from build123d import *

# Parameters (mm, degrees)
BOSS_EXTRUDE1_DEPTH = 50
SHELL1_T            = -1.5
SKETCH2_R           = 2.5
CUT_EXTRUDE1_DEPTH  = 50
SKETCH3_OUTSIDE_W   = 127.464
SKETCH3_OUTSIDE_H   = 87.464
CUT_EXTRUDE2_DEPTH  = 5
CUT_EXTRUDE2_TAPER  = 0.5
FILLET1_R           = 0.5
CHAMFER1_SIZE       = 1.25


with BuildPart() as part:
    # Sketch1 → Boss-Extrude1 (new body)
    with BuildSketch(Plane(origin=(0, 0, 0), x_dir=(1, 0, 0), z_dir=(0, 1, 0))):
        with BuildLine():
            Line((-47.5, -30), (47.5, -30))
            ThreePointArc((47.5, -30), (49.267766953, -29.267766953), (50, -27.5))
            Line((50, -27.5), (50, 27.5))
            ThreePointArc((50, 27.5), (49.267766953, 29.267766953), (47.5, 30))
            Line((47.5, 30), (-47.5, 30))
            ThreePointArc((-47.5, 30), (-49.267766953, 29.267766953), (-50, 27.5))
            Line((-50, 27.5), (-50, -27.5))
            ThreePointArc((-50, -27.5), (-49.267766953, -29.267766953), (-47.5, -30))
        make_face()
    extrude(amount=BOSS_EXTRUDE1_DEPTH)

    # Shell1
    shell1_openings = [part.faces().sort_by_distance(p)[0] for p in [
        (0, 50, 0),
    ]]
    offset(amount=SHELL1_T, openings=shell1_openings, kind=Kind.INTERSECTION)

    # Sketch2 → Cut-Extrude1 (cut)
    with BuildSketch(Plane(origin=(0, 1.5, 0), x_dir=(1, 0, 0), z_dir=(0, 1, 0))):
        with Locations((-40, 20)):
            Circle(SKETCH2_R)
        with Locations((40, 20)):
            Circle(SKETCH2_R)
        with Locations((40, -20)):
            Circle(SKETCH2_R)
        with Locations((-40, -20)):
            Circle(SKETCH2_R)
    extrude(amount=-CUT_EXTRUDE1_DEPTH, mode=Mode.SUBTRACT)

    # Sketch3 outside → Cut-Extrude2 (cut)
    with BuildSketch(Plane(origin=(0, 50, 0), x_dir=(1, 0, 0), z_dir=(0, 1, 0))):
        Rectangle(SKETCH3_OUTSIDE_W, SKETCH3_OUTSIDE_H)
        with BuildLine():
            Line((-47.767766953, -29.267766953), (47.767766953, -29.267766953))
            ThreePointArc((47.767766953, -29.267766953), (48.828427125, -28.828427125), (49.267766953, -27.767766953))
            Line((49.267766953, -27.767766953), (49.267766953, 27.767766953))
            ThreePointArc((49.267766953, 27.767766953), (48.828427125, 28.828427125), (47.767766953, 29.267766953))
            Line((47.767766953, 29.267766953), (-47.767766953, 29.267766953))
            ThreePointArc((-47.767766953, 29.267766953), (-48.828427125, 28.828427125), (-49.267766953, 27.767766953))
            Line((-49.267766953, 27.767766953), (-49.267766953, -27.767766953))
            ThreePointArc((-49.267766953, -27.767766953), (-48.828427125, -28.828427125), (-47.767766953, -29.267766953))
        make_face(mode=Mode.SUBTRACT)
    extrude(amount=-CUT_EXTRUDE2_DEPTH, taper=CUT_EXTRUDE2_TAPER, mode=Mode.SUBTRACT)

    # Fillet1
    fillet1_edges = [part.edges().sort_by_distance(p)[0] for p in [
        (-50, 0, 0),
        (-49.267766953, 0, -29.267766953),
        (0, 0, -30),
        (49.267766953, 0, -29.267766953),
        (50, 0, 0),
        (49.267766953, 0, 29.267766953),
        (0, 0, 30),
        (-49.267766953, 0, 29.267766953),
    ]]
    fillet(fillet1_edges, radius=FILLET1_R)

    # Chamfer1
    chamfer1_edges = [part.edges().sort_by_distance(p)[0] for p in [
        (-42.5, 1.5, -20),
        (37.5, 1.5, -20),
        (37.5, 1.5, 20),
        (-42.5, 1.5, 20),
    ]]
    chamfer(chamfer1_edges, length=CHAMFER1_SIZE)


solid = part.part
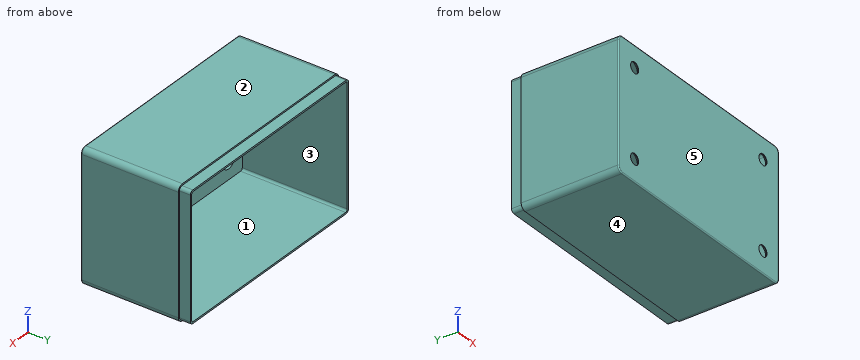
Read the model definition and answer for the solid it produces. Units are mm, in the model's axes. Face numbers are marked on the shaded views. A direction names the side the tool comes from. Give positions to 0.01 mm unless a question says otherwise; leave off trailing zeros. Loops run counter-clockwise (first coordinate to the right, second up) from the corner with the lowest first, then second, coordinate; pieces in that order, holes last. Notation, with made-up numbers: (50.25, -19.75) - (88.25, -19.75) arc R10 cw to (88.25, -1.75) - close; hole circle Ø4 at (38, -9). An arc over 180 degrees is marked (long way). Answer as CSV lines item,"result". Start each with the question number.
1) Which of the six approach directions +Z, -Z, +X, -X, +Y, -Y give full straight-line access (tool end or side, diameter ignored) to the marked faces 1 and 2?
2) Straight lines are drawn through the part: L1, parallel to X at y = 24.5, z = 23; L2, parallel to Z at x = 2, y = 28; L3, parallel to Z at x = 40, y = 0.1. For each, find the intervals that lie inside material, in ascending order. Write a range as from..to.
3) Find section B-B (x = -40). State how many separate pieces and enclosed holes the cut face has, then the cut area to 3 significant figures.
4) Find section A-A (y = 10). Write down the section's boundary in (x, z), then the cut area to 3 significant figures.
5) Determine the mould class of the marked faces 3, 4 and 5 for opening direction Z: released by +Z, released by -Z, zero draft, split by the parting line, or undercut.
6) Each of these flat-tipped pins is pushed along its axis until it touches: pin 1 Ø6.5 at (x, z) = (40, 20) entering from -Y; pin 2 Ø18 at (x, z) = (-9, -3.5) entering from +Y. Where does it stop, or does it pass through?
Findings below:
1,face 1,"+Y"
1,face 2,"+Z, +X, -X, +Y, -Y"
2,L1,"-50..-48.5, 48.5..50"
2,L2,"-30..-28.5, 28.5..30"
2,L3,"-29.8..-22.5, -17.5..17.5, 22.5..29.8"
3,separate pieces,"3"
3,enclosed holes,"0"
3,area,"210 mm^2"
4,outline,"(-50, -27.5) arc R2.5 ccw to (-47.5, -30) - (47.5, -30) arc R2.5 ccw to (50, -27.5) - (50, 27.5) arc R2.5 ccw to (47.5, 30) - (-47.5, 30) arc R2.5 ccw to (-50, 27.5) - close; hole (-48.5, -27.5) arc R1 ccw to (-47.5, -28.5) - (47.5, -28.5) arc R1 ccw to (48.5, -27.5) - (48.5, 27.5) arc R1 ccw to (47.5, 28.5) - (-47.5, 28.5) arc R1 ccw to (-48.5, 27.5) - close"
4,area,"466 mm^2"
5,face 3,"undercut"
5,face 4,"released by -Z"
5,face 5,"zero draft"
6,pin 1,"y = 0"
6,pin 2,"y = 1.5"
